Check sheet for the drawn part. Datum: minimum x, y, z corner. Units: mm. A direction names the side the tool comes from. Give positions to 0.01 mm unless a question says otherwise; leave off trailing zeros. Write each loop counter-clockwise with the first axis right and the second up, starting at its lowest first coordinate (ties: lowest second). Pieces come first, ordered by that corner, then holes. Notation, with made-up numbers: (57, 33) - (61, 33) arc R21 ccw to (61, 68) - close; hole circle Ø6 at (-22, -13.75). An arc over 180 degrees is marked (long way). Use a Markdown table: item, result.
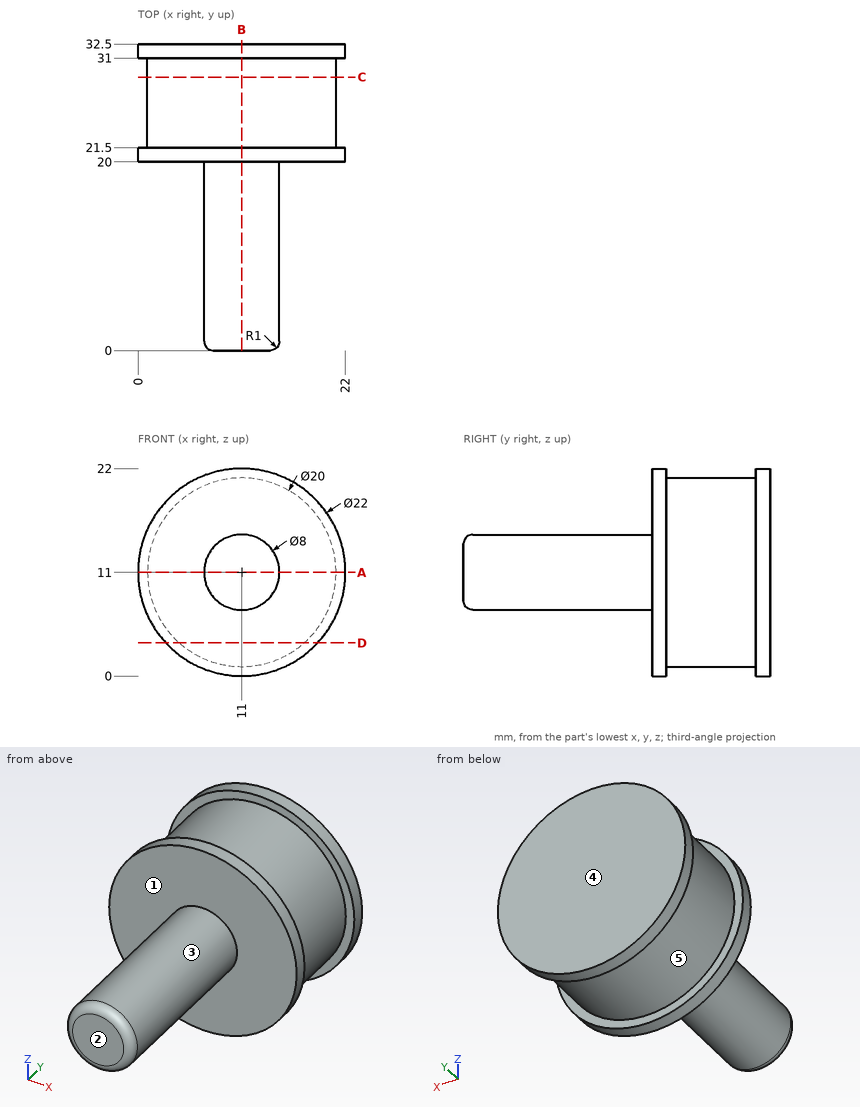
1) Set-up check for the marked faces 1 and 2: record each of +Z, -Z, +X, -X, +Y, -Y from which the full face is reachable in a straight line by a thin tool's end or side.
Working result:
| item | result |
|---|---|
| face 1 | -Y |
| face 2 | +Z, -Z, +X, -X, -Y |
2) Material ranges on L1, parallel to Y at x = 16, z = 2.25; L2, parallel to Y at x = 15.75, z = 8; L3, parallel to Z at x = 18.75, y = 22, recorded low to high. Write a range as from..to.
Working result:
| item | result |
|---|---|
| L1 | y = 20..21.5, 31..32.5 |
| L2 | y = 20..32.5 |
| L3 | z = 4.68..17.32 |
3) Section check D-D on z = 3.5. Record the boundary of the cut face in (x, y), then the cut area to 3 significant figures.
Working result:
| item | result |
|---|---|
| outline | (2.95, 20) - (19.05, 20) - (19.05, 21.5) - (17.61, 21.5) - (17.61, 31) - (19.05, 31) - (19.05, 32.5) - (2.95, 32.5) - (2.95, 31) - (4.39, 31) - (4.39, 21.5) - (2.95, 21.5) - close |
| area | 174 mm² |
4) Section check B-B on x = 11. Record the boundary of the cut face in (y, z).
Working result:
| item | result |
|---|---|
| outline | (0, 8) arc R1 ccw to (1, 7) - (20, 7) - (20, 0) - (21.5, 0) - (21.5, 1) - (31, 1) - (31, 0) - (32.5, 0) - (32.5, 22) - (31, 22) - (31, 21) - (21.5, 21) - (21.5, 22) - (20, 22) - (20, 15) - (1, 15) arc R1 ccw to (0, 14) - close |
5) Depth check by flat-ended pin: P1, Ø1, axis at x = 19, y = 21, coming from the +Z side; P2, Ø1, axis at y = 9, z = 14.5, coming from the +X side; P3, Ø5, axis at x = 19, y = 21.5, coming from the -Z side; P4, Ø6.5, axis at x = 12.5, z = 6, coming from the -Y side. Enter the tip coordinate at first touch or a pass-through.
Working result:
| item | result |
|---|---|
| P1 | stops at z = 19.05 |
| P2 | stops at x = 13.65 |
| P3 | stops at z = 1.47 |
| P4 | stops at y = 0 |
6) Section check C-C on y = 29. Record the boundary of the cut face in (x, z).
Working result:
| item | result |
|---|---|
| outline | circle Ø20 at (11, 11) |
7) Mould release check, pull along Y, two halves, no side actions. Record for the marked faces 3, 4 and 5: pulls with the +Y half, pulls with the -Y half, needs draft (parallel to the pull), parting line crosses it, or undercut.
Working result:
| item | result |
|---|---|
| face 3 | needs draft |
| face 4 | pulls with the +Y half |
| face 5 | undercut |
8) Section check A-A on z = 11. Record the boundary of the cut face in (x, y).
Working result:
| item | result |
|---|---|
| outline | (0, 20) - (7, 20) - (7, 1) arc R1 ccw to (8, 0) - (14, 0) arc R1 ccw to (15, 1) - (15, 20) - (22, 20) - (22, 21.5) - (21, 21.5) - (21, 31) - (22, 31) - (22, 32.5) - (0, 32.5) - (0, 31) - (1, 31) - (1, 21.5) - (0, 21.5) - close |
